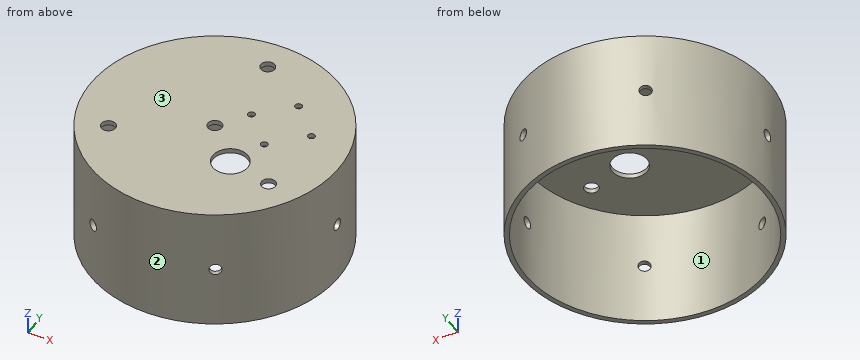
```python
from build123d import *

# Parameters (mm, degrees)
SKETCH1_R           = 53
BOSS_EXTRUDE1_DEPTH = 53
SKETCH2_R           = 3
CUT_EXTRUDE1_DEPTH  = 92.798692801
SHELL4_T            = -2
SKETCH6_R           = 1.5
CUT_EXTRUDE3_DEPTH  = 10
SKETCH7_R           = 7.5
CUT_EXTRUDE4_DEPTH  = 10
SKETCH8_R           = 51
CUT_EXTRUDE5_DEPTH  = 51
SKETCH9_R           = 2.5
CUT_EXTRUDE6_DEPTH  = 51
CIRPATTERN1_COUNT   = 6


with BuildPart() as part:
    # Sketch1 → Boss-Extrude1 (new body)
    with BuildSketch(Plane.XY):
        Circle(SKETCH1_R)
    extrude(amount=BOSS_EXTRUDE1_DEPTH)

    # Sketch2 → Cut-Extrude1 (cut, through all)
    with BuildSketch(Plane.XY.offset(53)):
        with Locations((0, 40)):
            Circle(SKETCH2_R)
        with Locations((34.641016151, -20)):
            Circle(SKETCH2_R)
        with Locations((-34.641016151, -20)):
            Circle(SKETCH2_R)
        Circle(SKETCH2_R)
    extrude(amount=-CUT_EXTRUDE1_DEPTH, mode=Mode.SUBTRACT)

    # Shell4
    shell4_openings = [part.faces().sort_by_distance(p)[0] for p in [
        (-51.500933624, 0, 0),
    ]]
    offset(amount=SHELL4_T, openings=shell4_openings, kind=Kind.INTERSECTION)

    # Sketch6 → Cut-Extrude3 (cut)
    with BuildSketch(Plane.XY.offset(53)):
        with Locations((21.650635095, 25.5)):
            Circle(SKETCH6_R)
        with Locations((34.650635095, 12.5)):
            Circle(SKETCH6_R)
        with Locations((21.650635095, -0.5)):
            Circle(SKETCH6_R)
        with Locations((8.650635095, 12.5)):
            Circle(SKETCH6_R)
    extrude(amount=-CUT_EXTRUDE3_DEPTH, mode=Mode.SUBTRACT)

    # Sketch7 → Cut-Extrude4 (cut)
    with BuildSketch(Plane.XY.offset(53)):
        with Locations((15.556349186, -15.556349186)):
            Circle(SKETCH7_R)
    extrude(amount=-CUT_EXTRUDE4_DEPTH, mode=Mode.SUBTRACT)

    # Sketch8 → Cut-Extrude5 (cut)
    with BuildSketch(Plane(origin=(0, 0, 0), x_dir=(-1, 0, 0), z_dir=(0, 0, -1))):
        with Locations(Location((0, 0, 0), (0, 0, 180))):
            Circle(SKETCH8_R)
    extrude(amount=-CUT_EXTRUDE5_DEPTH, mode=Mode.SUBTRACT)

    # Sketch9 → Cut-Extrude6 (cut)
    with BuildSketch(Plane.ZY.offset(53)):
        with Locations((26.5, 0)):
            Circle(SKETCH9_R)
    cut_extrude6 = extrude(amount=-CUT_EXTRUDE6_DEPTH, mode=Mode.SUBTRACT)

    # CirPattern1: Cut-Extrude6 ×6 about axis
    cirpattern1_axis = Axis((0, 0, 0), (0, 0, 1))
    for i in range(1, CIRPATTERN1_COUNT):
        add(cut_extrude6.rotate(cirpattern1_axis, i * 360 / CIRPATTERN1_COUNT), mode=Mode.SUBTRACT)


solid = part.part
```
Can you work these out from the model? Positions are in its coordinate system, mm. Face numbers are marked on the shaded views. Give positions to 0.01 mm unless a question says otherwise; leave off trailing zeros. Order: outer loops, then holes, each group sorted by start corner. A loop starts at its lowest first (then second) coordinate and runs counter-clockwise, first axis right, second up. Notation, with made-up numbers: (50, 43.5) - (69, 43.5) arc R11 ccw to (69, 56.5) - close; hole circle Ø6 at (61, 46). An arc over 180 degrees is marked (long way). Use a Markdown table: item, result. Add a question column.
Q1. I'm going to push flat-ended pins straight in: pin 1 (5 mm diameter, centred on x = 21.65, y = -0.5, fed in from -Z); pin 2 (4 mm diameter, centred on y = 14.5, z = 19, fed in from +X); pin 3 (4 mm diameter, centred on y = -28.5, z = 35, fed in from +X). Where does each tip first touch, or does it pass through?
Q2. If we section it at C-C on y = -20: Write out the boundary of the cut face in (x, z).
Q3. If we section it at D-D on y = 25.5: Write out the boundary of the cut face in (x, z).
Q4. If we mould it in two halves opening along X, with no side actions, what happens to the marked faces 1, 2 and 3? For each: released by +X, released by -X, zero draft, split by the parting line, or undercut.
Q5. If we section it at B-B on z = 26: Write out the boundary of the cut face in (x, y).
Q6. If we section it at A-A on x = 18: Write out the boundary of the cut face in (y, z), plus the area to 3 significant figures.
Q7. Please list where these lines run through material, in increasing order: line 1 along Y through (x, z) = (0, 52); line 2 along Z through (x, y) = (15, 16); line 3 along X through (y, z) = (-1, 15).
Answers follow:
| question | item | result |
|---|---|---|
| 1 | pin 1 | stops at z = 51 |
| 1 | pin 2 | stops at x = 51.5 |
| 1 | pin 3 | stops at x = 45.9 |
| 2 | outline | (-49.08, 0) - (-46.91, 0) - (-46.91, 51) - (-37.64, 51) - (-37.64, 53) - (-49.08, 53) - close; (-31.64, 51) - (9.51, 51) - (9.51, 53) - (-31.64, 53) - close; (21.6, 51) - (31.64, 51) - (31.64, 53) - (21.6, 53) - close; (37.64, 51) - (46.91, 51) - (46.91, 0) - (49.08, 0) - (49.08, 53) - (37.64, 53) - close |
| 3 | outline | (-46.46, 0) - (-44.17, 0) - (-44.17, 51) - (20.15, 51) - (20.15, 53) - (-46.46, 53) - close; (23.15, 51) - (44.17, 51) - (44.17, 0) - (46.46, 0) - (46.46, 53) - (23.15, 53) - close |
| 4 | face 1 | undercut |
| 4 | face 2 | split by the parting line |
| 4 | face 3 | zero draft |
| 5 | outline | (-52.94, -2.45) arc R53 ccw to (-28.59, -44.63) - (-27.59, -42.89) arc R51 cw to (-50.94, -2.45) - close; (-52.94, 2.45) - (-50.94, 2.45) arc R51 cw to (-27.59, 42.89) - (-28.59, 44.63) arc R53 ccw to start; (-24.35, -47.08) arc R53 ccw to (24.35, -47.08) - (23.35, -45.34) arc R51 cw to (-23.35, -45.34) - close; (-24.35, 47.08) - (-23.35, 45.34) arc R51 cw to (23.35, 45.34) - (24.35, 47.08) arc R53 ccw to start; (27.59, -42.89) - (28.59, -44.63) arc R53 ccw to (52.94, -2.45) - (50.94, -2.45) arc R51 cw to start; (27.59, 42.89) arc R51 cw to (50.94, 2.45) - (52.94, 2.45) arc R53 ccw to (28.59, 44.63) - close |
| 6 | outline | (-49.85, 0) - (-47.72, 0) - (-47.72, 51) - (-22.65, 51) - (-22.65, 53) - (-49.85, 53) - close; (-8.47, 51) - (47.72, 51) - (47.72, 0) - (49.85, 0) - (49.85, 53) - (-8.47, 53) - close |
| 6 | area | 388 mm^2 |
| 7 | line 1 | y = -53 to -3, 3 to 37, 43 to 53 |
| 7 | line 2 | z = 51 to 53 |
| 7 | line 3 | x = -52.99 to -50.99, 50.99 to 52.99 |
